Could you check a few things on this model? Use its own coordinates, in mm. A direction names the side the tool comes from. Round coordinates to 2 decimals unless told otherwise and drop trailing zeros. Write each loop counter-clockwise with the first axis right and the second up, starting at its lowest first coordinate (ties: lowest second). Pieces come first, ordered by that corner, then holes. Notation, with made-up numbers: (-6, 37) -> (46, 37) arc R20 ccw to (46, 65) -> close; hole circle Ø6 at (-19.75, 1.25). An arc over 180 degrees is marked (long way). Answer in a Markdown table with one row per item. Add a question column.
```python
from build123d import *

# Parameters (mm, degrees)
SKETCH2_R           = 9
SKETCH2_R_2         = 6
BOSS_EXTRUDE1_DEPTH = 4
CHAMFER2_SIZE       = 0.25
SKETCH3_R           = 8
SKETCH3_R_2         = 7
CUT_EXTRUDE2_DEPTH  = 0.5
SKETCH4_R           = 8
SKETCH4_R_2         = 7
CUT_EXTRUDE3_DEPTH  = 0.5
CHAMFER3_SIZE       = 0.25


with BuildPart() as part:
    # Sketch2 → Boss-Extrude1 (new body)
    with BuildSketch(Plane.XY):
        Circle(SKETCH2_R)
        Circle(SKETCH2_R_2, mode=Mode.SUBTRACT)
    extrude(amount=BOSS_EXTRUDE1_DEPTH)

    # Chamfer2
    chamfer2_edges = [part.edges().sort_by_distance(p)[0] for p in [
        (-9, 0, 0),
        (-9, 0, 4),
        (-6, 0, 0),
        (-6, 0, 4),
    ]]
    chamfer(chamfer2_edges, length=CHAMFER2_SIZE)

    # Sketch3 → Cut-Extrude2 (cut)
    with BuildSketch(Plane(origin=(0, 0, 0), x_dir=(-1, 0, 0), z_dir=(0, 0, -1))):
        Circle(SKETCH3_R)
        Circle(SKETCH3_R_2, mode=Mode.SUBTRACT)
    extrude(amount=-CUT_EXTRUDE2_DEPTH, mode=Mode.SUBTRACT)

    # Sketch4 → Cut-Extrude3 (cut)
    with BuildSketch(Plane.XY.offset(4)):
        Circle(SKETCH4_R)
        Circle(SKETCH4_R_2, mode=Mode.SUBTRACT)
    extrude(amount=-CUT_EXTRUDE3_DEPTH, mode=Mode.SUBTRACT)

    # Chamfer3
    chamfer3_edges = [part.edges().sort_by_distance(p)[0] for p in [
        (8, 0, 0),
        (7, 0, 0),
        (-8, 0, 4),
        (-7, 0, 4),
    ]]
    chamfer(chamfer3_edges, length=CHAMFER3_SIZE)


solid = part.part
```
(1) Suppose I cut it at A-A, the plane z = 0.75. Please give me the cut outline in (x, y).
(2) If we mould it in two halves opening along X, with no side actions, what happens to faces 1 (the face through (-1.172, 8.923, 1.976)), 2 (the face through (5, -4, 0)), 3 (the face through (-4, -6, 0.5))? For each: pulls with the +X half, pulls with the -X half, needs draft (parallel to the pull), parting line crosses it, or undercut.
(3) On a 3-axis mill with a long thin cutter (end or side, diameter ignored), from which of +Z, -Z, +X, -X, +Y, -Y can I reach the whole of each face in a straight line? I mean faces 4 (the face through (-8, 3, 0)), 5 (the face through (4, -6, 3.5)). Say none if no direction works.
(4) For P1, Ø1, axis at x = -2.5, z = 2, coming from the -Y side; P2, Ø2, axis at y = -6.5, z = 2, coming from the +X side; P3, Ø1, axis at y = -7, z = 2.5, coming from the -X side, each with a flat end and sliding along its axis, tell me the tip position at first contact or that it passes through.
(5) I need wall thicknesses on L1, parallel to Y at x = 0, z = 3.65; L2, parallel to Y at x = 0, z = 1.2; L3, parallel to X at y = -5.5, z = 2.1. Which ranges of each line are inside material? Lowest first, please.
Response:
| question | item | result |
|---|---|---|
| 1 | outline | circle Ø18 at (0, 0); hole circle Ø12 at (0, 0) |
| 2 | face 1 | parting line crosses it |
| 2 | face 2 | needs draft |
| 2 | face 3 | undercut |
| 3 | face 4 | -Z, +X, -X, +Y, -Y |
| 3 | face 5 | +Z |
| 4 | P1 | y = -8.77 |
| 4 | P2 | x = 7.12 |
| 4 | P3 | x = -6.22 |
| 5 | L1 | -9 to -8, -7 to -6, 6 to 7, 8 to 9 |
| 5 | L2 | -9 to -6, 6 to 9 |
| 5 | L3 | -7.12 to -2.4, 2.4 to 7.12 |
